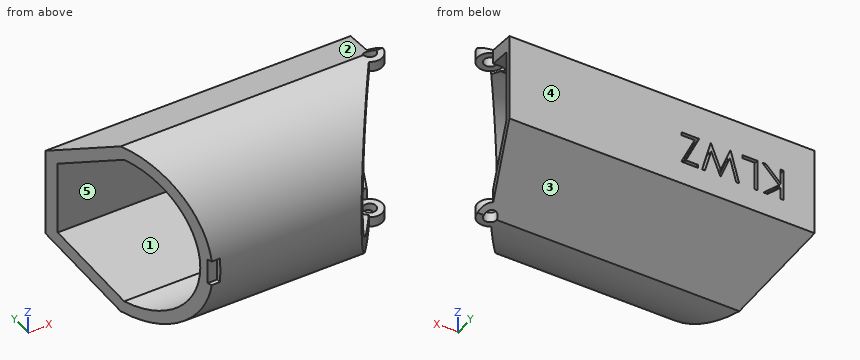
from build123d import *

# Parameters (mm, degrees)
BOSS_EXTRUDE1_DEPTH     = 30.48
SHELL1_T                = -1.27
SKETCH2_R               = 0.635
CUT_EXTRUDE1_DEPTH      = 9.904502457
CUT_EXTRUDE1_DEPTH_BACK = 9.904502457
SKETCH4_R               = 1.27
CUT_EXTRUDE3_DEPTH      = 7.874
CUT_EXTRUDE3_DEPTH_BACK = 7.874
SKETCH5_W               = 1.524
SKETCH5_H               = 2.54
CUT_EXTRUDE5_DEPTH      = 0.508
CUT_EXTRUDE2_DEPTH      = 0.762


with BuildPart() as part:
    # Sketch1 → Boss-Extrude1 (new body)
    with BuildSketch(Plane(origin=(0, 0, 0), x_dir=(0, 0, -1), z_dir=(1, 0, 0))):
        with BuildLine():
            Line((-4.445, 0), (4.445, 0))
            Line((4.445, 0), (8.89, -7.69896584))
            ThreePointArc((8.89, -7.69896584), (0, -17.111468296), (-8.89, -7.69896584))
            Line((-8.89, -7.69896584), (-4.445, 0))
        make_face()
    extrude(amount=BOSS_EXTRUDE1_DEPTH)

    # Shell1
    shell1_openings = [part.faces().sort_by_distance(p)[0] for p in [
        (30.48, -6.202608534, 0),
        (0, -6.202608534, 0),
    ]]
    offset(amount=SHELL1_T, openings=shell1_openings, kind=Kind.INTERSECTION)

    # Sketch2 → Cut-Extrude1 (cut, two sides)
    with BuildSketch(Plane.XY) as cut_extrude1_sk:
        with Locations((27.6778056, -7.69896584)):
            Circle(SKETCH2_R)
        with BuildLine():
            Line((30.48, 0), (28.112171182, -6.505556211))
            ThreePointArc((28.112171182, -6.505556211), (28.804309358, -8.285386578), (26.949363526, -8.739288936))
            Line((26.949363526, -8.739288936), (21.087100426, -17.111468296))
            Line((21.087100426, -17.111468296), (30.48, -17.111468296))
            Line((30.48, -17.111468296), (30.48, 0))
        make_face()
        Polygon((0, 0), (6.228065124, -17.111468296), (0, -17.111468296), align=None)
    extrude(amount=CUT_EXTRUDE1_DEPTH, mode=Mode.SUBTRACT)
    extrude(cut_extrude1_sk.sketch, amount=-CUT_EXTRUDE1_DEPTH_BACK, mode=Mode.SUBTRACT)

    # Sketch4 → Cut-Extrude3 (cut, two sides)
    with BuildSketch(Plane.XY) as cut_extrude3_sk:
        with Locations((27.6778056, -7.69896584)):
            Circle(SKETCH4_R)
    extrude(amount=CUT_EXTRUDE3_DEPTH, mode=Mode.SUBTRACT)
    extrude(cut_extrude3_sk.sketch, amount=-CUT_EXTRUDE3_DEPTH_BACK, mode=Mode.SUBTRACT)

    # Sketch5 → Cut-Extrude5 (cut)
    with BuildSketch(Plane(origin=(0, -17.111468296, 0), x_dir=(1, 0, 0), z_dir=(0, 1, 0))):
        with Locations((6.228065124, 0)):
            Rectangle(SKETCH5_W, SKETCH5_H)
    extrude(amount=CUT_EXTRUDE5_DEPTH, mode=Mode.SUBTRACT)

    # Sketch3 → Cut-Extrude2 (cut)
    with BuildSketch(Plane(origin=(0, 0, 0), x_dir=(1, 0, 0), z_dir=(0, 1, 0))):
        Polygon((3.102574475, 2.126725666), (3.387510372, 2.126725666), (3.387510372, 0.917656155), (4.711063057, 2.126725666), (5.117478321, 2.126725666), (3.557327079, 0.702046179), (5.239593706, -1.048274334), (4.859891182, -1.048274334), (3.387510372, 0.483892132), (3.387510372, -1.048274334), (3.102574475, -1.048274334), align=None)
        Polygon((5.70770268, 2.126725666), (5.992638577, 2.126725666), (5.992638577, -0.722633308), (7.213792424, -0.722633308), (7.213792424, -1.048274334), (5.70770268, -1.048274334), align=None)
        Polygon((7.539433449, 2.126725666), (7.833909611, 2.126725666), (8.455298834, -0.201734871), (9.379432448, 2.126725666), (9.420773594, 2.126725666), (10.327734731, -0.18583443), (10.952304042, 2.126725666), (11.243600116, 2.126725666), (10.387520388, -1.048274334), (10.34681526, -1.048274334), (9.391516783, 1.380040971), (8.424769988, -1.048274334), (8.38406486, -1.048274334), align=None)
        Polygon((11.650651398, 1.80108464), (11.650651398, 2.126725666), (13.319561654, 2.126725666), (11.987740741, -0.722633308), (13.278856526, -0.722633308), (13.278856526, -1.048274334), (11.528536013, -1.048274334), (12.860356927, 1.80108464), align=None)
    extrude(amount=-CUT_EXTRUDE2_DEPTH, mode=Mode.SUBTRACT)


solid = part.part
Could you check a few things on this model? Use its own coordinates, in mm. Face numbers are marked on the shaded views. A direction names the side the tool comes from. Give positions to 0.01 mm unless a question says otherwise; leave off trailing zeros. Order: outer loops, then holes, each group sorted by start corner. A loop starts at its lowest first (then second) coordinate and runs counter-clockwise, first axis right, second up.
Item 1: For the marked faces 4 and 5, which set-ups out of +Z, -Z, +X, -X, +Y, -Y let a thin tool reach every point of the face, with its end or its side?
Item 2: I need wall thicknesses on line 1 (Z direction, x = 15, y = -7.5); line 2 (Z direction, x = 25, y = -1.75); line 3 (Y direction, x = 6.5, z = -2). Which ranges of each line are inside material? Lowest first, please.
Item 3: If we section it at A-A, the plane x = 17.5: Write out the boundary of the cut face in (y, z) (1 decimal).
Item 4: I'm going to push flat-ended pins straight in: pin 1 (1 mm diameter, centred on x = 16.5, z = 6, fed in from -Y); pin 2 (3 mm diameter, centred on x = 27.5, y = -8, fed in from -Z); pin 3 (4 mm diameter, centred on x = 13.5, z = -4.5, fed in from -Y); pin 4 (4 mm diameter, centred on x = 9.5, z = 3.5, fed in from -Y). Where does each tip first touch, or does it pass through?
Item 5: If we section it at C-C, the plane y = -15: Write out the boundary of the cut face in (x, z).
Item 6: If we mould it in two halves opening along Z, with no side actions, what happens to the marked faces 1, 2 and 3? For each: pulls with the +Z half, pulls with the -Z half, needs draft (parallel to the pull), parting line crosses it, or undercut.
Item 7: If we section it at B-B, the plane y = -10.75: Write out the boundary of the cut face in (x, z).
Values:
1. face 4: +Z, -Z, +X, -X, +Y
1. face 5: +X, -X
2. line 1: z = -8.78 to -7.31, 7.31 to 8.78
2. line 2: z = -5.46 to -3.99, 3.99 to 5.46
2. line 3: y = -16.88 to -15.57, -1.27 to 0
3. outline: (-7.7, -8.9) - (0, -4.4) - (0, 4.4) - (-7.7, 8.9) arc R8.9 ccw (long way) to start; hole (-8.1, -7.6) - (-1.3, -3.7) - (-1.3, 3.7) - (-8.1, 7.6) arc R7.6 ccw (long way) to start
4. pin 1: stops at y = -15.21
4. pin 2: stops at z = -8.9
4. pin 3: stops at y = -16.75
4. pin 4: stops at y = -16.98
5. outline: (5.46, -5.76) - (22.57, -5.76) - (22.57, -3.48) - (5.46, -3.48) - close; (5.46, 3.48) - (22.57, 3.48) - (22.57, 5.76) - (5.46, 5.76) - close
6. face 1: undercut
6. face 2: pulls with the +Z half
6. face 3: pulls with the -Z half
7. outline: (3.91, -8.53) - (25.54, -8.53) - (25.54, -7.2) - (3.91, -7.2) - close; (3.91, 7.2) - (25.54, 7.2) - (25.54, 8.53) - (3.91, 8.53) - close
